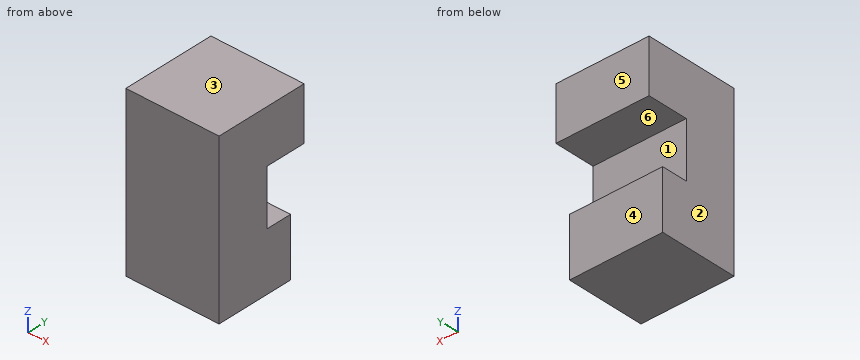
Autodesk Inventor part; units mm, degrees
ref_plane "YZ Plane" through (0, 0, 0) normal (1, 0, 0) x (0, 1, 0)
ref_plane "XZ Plane" through (0, 0, 0) normal (0, 1, 0) x (-1, 0, 0)
ref_plane "XY Plane" through (0, 0, 0) normal (0, 0, 1) x (1, 0, 0)
sketch "Esboço1" plane through (0, 0, 0) normal (1, 0, 0) x (0, 1, 0)
  line L0 (0, 0) -> (25, 0)
  line L1 (25, 0) -> (25, -45)
  line L2 (25, -45) -> (0, -45)
  line L3 (0, -45) -> (0, 0)
  dimension "d0" = 45
  dimension "d1" = 25
extrude "Extrusão1" add sketch "Esboço1" along normal blind 25
sketch "Esboço4" plane through (0, 0, 0) normal (-1, 0, 0) x (0, 0, 1)
  line L0 (-29.275, 25) -> (-14.275, 25)
  line L1 (-14.275, 25) -> (-14.275, 14.0681)
  line L2 (-14.275, 14.0681) -> (-29.275, 14.0681)
  line L3 (-29.275, 14.0681) -> (-29.275, 25)
  line L4 (0, 0) -> (-45, 0)
  dimension "d8" = 25
  dimension "d9" = 15
extrude "Extrusão3" cut sketch "Esboço4" against normal through all
sketch "Esboço6" plane through (0, 0, 0) normal (-1, 0, 0) x (0, 0, 1)
  line L0 (-45, 25) -> (-29.275, 25)
  line L1 (-29.275, 14.0681) -> (-29.275, 25)
  line L2 (-45, 25) -> (-29.275, 25)
  line L3 (-29.275, 25) -> (-29.275, 21)
  line L4 (-29.275, 21) -> (-45, 21)
  line L5 (-45, 21) -> (-45, 25)
  point P0 (0, 0)
  point P1 (-37.1375, 21)
  dimension "d12" = 4
  dimension "d13" = 15.725
extrude "Extrusão4" cut sketch "Esboço6" against normal through all
properties part number "Peça2_aula"
Can you work these out from the model? Positions are in its coordinate system, mm. Face numbers are marked on the shaded views. A direction names the side the tool comes from. Round coordinates to 2 decimals unless told otherwise and drop trailing zeros. Loops run counter-clockwise (first coordinate to the right, second up) from the corner with the lowest first, then second, coordinate; pieces in that order, holes last. Notation, with made-up numbers: M -29.75,-39.75 L -1.75,-39.75 A7 cw -1.75,-34.75 Z; hole C 16.5,-7 d9. An arc over 180 degrees is marked long. Write item = value, one per line. Start each with the question number.
(1) I need wall thicknesses on line 1 along Z through (x, y) = (7.25, 14.25) (3 decimals); line 2 along Z through (x, y) = (20, 24) (3 decimals); line 3 along Y through (x, z) = (15, -27). Which ranges of each line are inside material? Lowest first, please.
(2) Suppose I cut it at B-B on x = 3.5. Write out the boundary of the cut face in (y, z) (3 decimals).
(3) I'm going to push flat-ended pins straight in: P1, Ø1, axis at x = 10.5, y = 9, coming from the +Z side; P2, Ø7.5, axis at x = 9.5, z = -19, coming from the +Y side; P3, Ø4.5, axis at x = 9.5, z = -33.5, coming from the +Y side. Where does each tip first touch, or does it pass through?
(4) Which directions (+Z, -Z, +X, -X, +Y, -Y) give clear straight access to the entire face, cutting with the end or side of a thin tool? Please do the marked faces 4, 5 and 6.
(5) If we mould it in two halves opening along Z, with no side actions, what happens to the marked faces 1, 2 and 3? For each: released by +Z, released by -Z, zero draft, split by the parting line, or undercut.
(6) Suppose I cut it at C-C on z = -15. Write out the boundary of the cut face in (x, y).
(7) Suppose I cut it at A-A on y = 16.75. Write out the boundary of the cut face in (x, z) (3 decimals), plus the area to 3 significant figures.
(8) Suppose I cut it at D-D on z = -35. Write out the boundary of the cut face in (x, y), plus the area to 3 significant figures.
Answer block:
q1.line_1 = -45 to -29.275, -14.275 to 0
q1.line_2 = -14.275 to 0
q1.line_3 = 0 to 14.07
q2.outline = M 0,-45 L 21,-45 L 21,-29.275 L 14.068,-29.275 L 14.068,-14.275 L 25,-14.275 L 25,0 L 0,0 Z
q3.P1 = 0
q3.P2 = 14.07
q3.P3 = 21
q4.face_4 = -Z, +X, -X, +Y
q4.face_5 = +Z, -Z, +X, -X, +Y
q4.face_6 = +X, -X, +Y
q5.face_1 = undercut
q5.face_2 = zero draft
q5.face_3 = released by +Z
q6.outline = M 0,0 L 25,0 L 25,14.07 L 0,14.07 Z
q7.outline = M 0,-45 L 25,-45 L 25,-29.275 L 0,-29.275 Z; M 0,-14.275 L 25,-14.275 L 25,0 L 0,0 Z
q7.area = 750 mm²
q8.outline = M 0,0 L 25,0 L 25,21 L 0,21 Z
q8.area = 525 mm²
